Input: part model. Units: mm. Frame: model coordinates. Give positions to 0.01 mm unless a question says otherwise; leave off trailing zeros. Write each loop counter-clockwise with the first axis right and the second up, starting at its lowest first coordinate (ties: lowest second). Pieces come first, ordered by that corner, then holes. Notation, with made-up numbers: (-18, 10) - (12, 10) arc R24 cw to (12, 25) - close; hole circle Ø7 at (-29.75, -30.5). An arc over 180 degrees is marked (long way). Answer as a JSON object with one key per item and string values. Group by question number.
from build123d import *
from build123d.topology import SkipClean

# Parameters (mm, degrees)
BOSS_EXTRUDE1_DEPTH             = 177.8
BOSS_EXTRUDE1_2_DEPTH           = 177.8
SKETCH2_R                       = 63.5
SKETCH2_R_2                     = 61.9125
BOSS_EXTRUDE2_DEPTH             = 101.6
BOSS_EXTRUDE3_START             = -12.7
SKETCH3_R                       = 61.9125
SKETCH3_R_2                     = 31.75
BOSS_EXTRUDE3_DEPTH             = 12.7
F_1_4_0_25_DIAMETER_HOLE1_D     = 6.35
F_1_4_0_25_DIAMETER_HOLE1_DEPTH = 44.958
CUT_EXTRUDE1_START              = -44.4500001
CUT_EXTRUDE1_DEPTH              = 32.0675001
BOSS_EXTRUDE6_REACH             = 449.258
SKETCH7_W                       = 15.24
SKETCH7_H                       = 7.62
SKETCH8_R                       = 2.54
CUT_EXTRUDE2_DEPTH              = 5.08


# Read off the part's stored shape, not the designer's step: Cut-Extrude1
with BuildPart() as part:
    # Sketch1 → Boss-Extrude1 (new, symmetric)
    with BuildSketch(Plane.XY):
        with BuildLine():
            ThreePointArc((60.57513929, 19.05), (0, 63.5), (-60.57513929, 19.05))
            Line((-60.57513929, 19.05), (-58.908871626, 19.05))
            ThreePointArc((-58.908871626, 19.05), (0, 61.9125), (58.908871626, 19.05))
            Line((58.908871626, 19.05), (60.57513929, 19.05))
        make_face()
    extrude(amount=BOSS_EXTRUDE1_DEPTH, both=True)



with BuildPart() as body_2:
    # Sketch1 → Boss-Extrude1 2 (new, symmetric)
    with BuildSketch(Plane.XY):
        with BuildLine():
            Line((-58.908871626, -19.05), (-60.57513929, -19.05))
            ThreePointArc((-60.57513929, -19.05), (0, -63.5), (60.57513929, -19.05))
            Line((60.57513929, -19.05), (58.908871626, -19.05))
            ThreePointArc((58.908871626, -19.05), (0, -61.9125), (-58.908871626, -19.05))
        make_face()
    extrude(amount=BOSS_EXTRUDE1_2_DEPTH, both=True)


with BuildPart() as part_1:
    with SkipClean():  # the faces are left unmerged after this step: merging them gives an invalid solid
        add(part.part)

        add(body_2.part)  # Boss-Extrude2 merges body 2
        # Sketch2 → Boss-Extrude2 (add)
        with BuildSketch(Plane(origin=(0, 0, -177.8), x_dir=(-1, 0, 0), z_dir=(0, 0, -1))):
            Circle(SKETCH2_R)
            Circle(SKETCH2_R_2, mode=Mode.SUBTRACT)
        extrude(amount=BOSS_EXTRUDE2_DEPTH)

    # Sketch3 → Boss-Extrude3 (add)
    with SkipClean():  # the faces are left unmerged after this step: merging them gives an invalid solid
        with BuildSketch(Plane(origin=(0, 0, -273.05), x_dir=(-1, 0, 0), z_dir=(0, 0, -1)).offset(BOSS_EXTRUDE3_START)):
            Circle(SKETCH3_R)
            Circle(SKETCH3_R_2, mode=Mode.SUBTRACT)
        extrude(amount=BOSS_EXTRUDE3_DEPTH)

    # 1/4 (0.25) Diameter Hole1
    with Locations(Plane(origin=(0, 44.45, -273.05), x_dir=(-1, 0, 0), z_dir=(0, 0, -1))):
        with Locations((0, 0), (44.45, -44.45), (0, -88.9), (-44.45, -44.45)):
            Hole(F_1_4_0_25_DIAMETER_HOLE1_D / 2, depth=F_1_4_0_25_DIAMETER_HOLE1_DEPTH)

    # Cut-Extrude1 outline → Cut-Extrude1 (cut)
    with BuildSketch(Plane(origin=(0, -19.05, 0), x_dir=(1, 0, 0), z_dir=(0, 1, 0)).offset(CUT_EXTRUDE1_START)):
        Polygon((-53.34, 219.71), (-38.1, 219.71), (-38.1, -3.81), (-53.34, -3.81), (-53.34, -19.05), (-38.1, -19.05), (-38.1, -44.45), (38.1, -44.45), (38.1, -19.05), (53.34, -19.05), (53.34, -3.81), (38.1, -3.81), (38.1, 219.71), (53.34, 219.71), (53.34, 234.95), (38.1, 234.95), (38.1, 260.35), (-38.1, 260.35), (-38.1, 234.95), (-53.34, 234.95), align=None)
    extrude(amount=CUT_EXTRUDE1_DEPTH, mode=Mode.SUBTRACT)

    # Boss-Extrude6: up to this face of the body (flat: up to its plane)
    boss_extrude6_end = Plane(part_1.part.faces().sort_by_distance((-46.232796628, -41.83821412, 19.05))[0])
    # Sketch7 → Boss-Extrude6 (add, up to the picked face)
    with BuildSketch(Plane.XY.offset(-260.35), mode=Mode.PRIVATE) as boss_extrude6_sk1:
        with BuildLine():
            ThreePointArc((53.34, -31.4325), (55.376223463, -27.688111731), (57.15, -23.8125))
            Line((57.15, -23.8125), (53.34, -23.8125))
            Line((53.34, -23.8125), (53.34, -31.4325))
        make_face()
    boss_extrude6_tool1 = split(extrude(boss_extrude6_sk1.sketch, amount=BOSS_EXTRUDE6_REACH, mode=Mode.PRIVATE), bisect_by=boss_extrude6_end, keep=Keep.BOTH, mode=Mode.PRIVATE)
    # Sketch7 → Boss-Extrude6 (add, up to the picked face)
    with BuildSketch(Plane.XY.offset(-260.35), mode=Mode.PRIVATE) as boss_extrude6_sk2:
        with Locations((45.72, -27.6225)):
            Rectangle(SKETCH7_W, SKETCH7_H)
    boss_extrude6_tool2 = split(extrude(boss_extrude6_sk2.sketch, amount=BOSS_EXTRUDE6_REACH, mode=Mode.PRIVATE), bisect_by=boss_extrude6_end, keep=Keep.BOTH, mode=Mode.PRIVATE)
    # Sketch7 → Boss-Extrude6 (add, up to the picked face)
    with BuildSketch(Plane.XY.offset(-260.35), mode=Mode.PRIVATE) as boss_extrude6_sk3:
        with BuildLine():
            Line((-53.34, -31.4325), (-53.34, -23.8125))
            Line((-53.34, -23.8125), (-57.15, -23.8125))
            ThreePointArc((-57.15, -23.8125), (-55.376223463, -27.688111731), (-53.34, -31.4325))
        make_face()
    boss_extrude6_tool3 = split(extrude(boss_extrude6_sk3.sketch, amount=BOSS_EXTRUDE6_REACH, mode=Mode.PRIVATE), bisect_by=boss_extrude6_end, keep=Keep.BOTH, mode=Mode.PRIVATE)
    # Sketch7 → Boss-Extrude6 (add, up to the picked face)
    with BuildSketch(Plane.XY.offset(-260.35), mode=Mode.PRIVATE) as boss_extrude6_sk4:
        with Locations((-45.72, -27.6225)):
            Rectangle(SKETCH7_W, SKETCH7_H)
    boss_extrude6_tool4 = split(extrude(boss_extrude6_sk4.sketch, amount=BOSS_EXTRUDE6_REACH, mode=Mode.PRIVATE), bisect_by=boss_extrude6_end, keep=Keep.BOTH, mode=Mode.PRIVATE)
    add(boss_extrude6_tool1.solids().sort_by(Axis((54.64733, -26.422885, -260.35), (0, 0, 1)))[0])
    add(boss_extrude6_tool2.solids().sort_by(Axis((45.72, -27.6225, -260.35), (0, 0, 1)))[0])
    add(boss_extrude6_tool3.solids().sort_by(Axis((-54.64733, -26.422885, -260.35), (0, 0, 1)))[0])
    add(boss_extrude6_tool4.solids().sort_by(Axis((-45.72, -27.6225, -260.35), (0, 0, 1)))[0])

    # Sketch8 → Cut-Extrude2 (cut)
    with SkipClean():  # the faces are left unmerged after this step: merging them gives an invalid solid
        with BuildSketch(Plane.XZ.offset(31.4325)):
            with Locations((-45.72, 11.352572264)):
                Circle(SKETCH8_R)
            with Locations((-45.72, -227.33)):
                Circle(SKETCH8_R)
            with Locations(Location((45.72, 11.352572264, 0), (0, 0, 180))):
                Circle(SKETCH8_R)
            with Locations(Location((45.72, -227.33, 0), (0, 0, 180))):
                Circle(SKETCH8_R)
        extrude(amount=-CUT_EXTRUDE2_DEPTH, mode=Mode.SUBTRACT)


solid = part_1.part
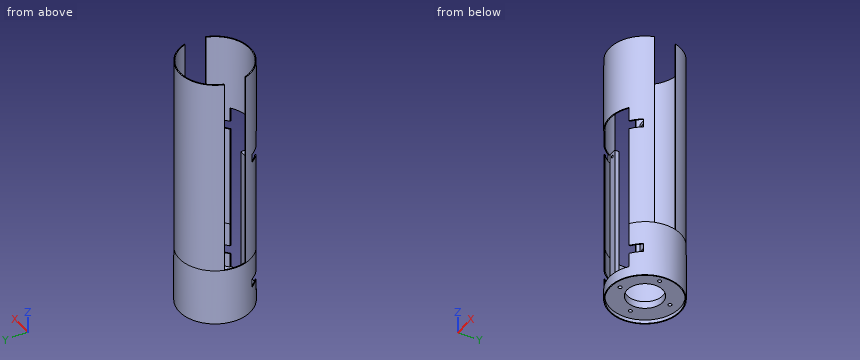
1) Line query: line 1 along Y through (x, z) = (0, -266.5) (3 decimals); line 2 along Z through (x, y) = (-45.72, -29.4); line 3 along Y through (x, z) = (-47, -236.5). Output: solid intervals per line, ascending. Write a range as from..to.
2) Pin query (flat end, axial travel): P1, Ø4, axis at y = -51, z = 94, coming from the +X side; P2, Ø5, axis at x = -36, y = -33.5, coming from the -Z side; P3, Ø6, axis at x = 48.5, z = 64, coming from the +Y side; P4, Ø2, axis at y = 16.5, z = 105.5, coming from the +X side. Return the tip coordinate at first contact, or that it passes through.
3) Cut plane A-A on z = -156. Count the separate pieces of the cut face and the enclosed holes in it, and give its area (3 significant figures).
4) Cut plane C-C on x = -8. Return the cut outline in (y, z).
Filled in:
{
 "1": {"line 1": "y = -63.5..-47.625, -41.275..-31.75, 31.75..41.275, 47.625..63.5", "line 2": "z = -273.05..-229.87, -224.79..8.81, 13.89..19.05", "line 3": "y = -42.7..-40.3, -31.43..-23.81, 40.3..42.7"},
 "2": {"P1": "stops at x = 40.39", "P2": "stops at z = -273.05", "P3": "stops at y = 44.29", "P4": "passes through"},
 "3": {"separate pieces": "3", "enclosed holes": "0", "area": "635 mm²"},
 "4": {"outline": "(-62.99, -279.4) - (-61.39, -279.4) - (-61.39, -273.05) - (-30.73, -273.05) - (-30.73, -260.35) - (-62.99, -260.35) - close; (-62.99, 44.45) - (-61.39, 44.45) - (-61.39, 177.8) - (-62.99, 177.8) - close; (30.73, -273.05) - (61.39, -273.05) - (61.39, -279.4) - (62.99, -279.4) - (62.99, 177.8) - (61.39, 177.8) - (61.39, -260.35) - (30.73, -260.35) - close"}
}
